```python
from build123d import *

# Parameters (mm, degrees)
F0_W     = 127
F0_H     = 127
F1_DEPTH = 12.7
F2_R     = 12.7
F3_DEPTH = 6.35
F4_R     = 1.5875
F5_DEPTH = 6.351


with BuildPart() as f1:
    # F0 (on Front) → F1 (new body)
    with BuildSketch(Plane.XZ):
        Rectangle(F0_W, F0_H)
    extrude(amount=F1_DEPTH)

    # F2 (on face) → F3 (cut)
    with BuildSketch(Plane.XZ.offset(12.7)):
        with Locations((0, 34.29)):
            Circle(F2_R)
        with Locations((-29.696011, -17.145)):
            Circle(F2_R)
        with Locations((29.696011, -17.145)):
            Circle(F2_R)
    extrude(amount=-F3_DEPTH, mode=Mode.SUBTRACT)

    # F4 (on face) → F5 (cut, through all)
    with BuildSketch(Plane.XZ.offset(6.35)):
        with Locations((0, 45.4025)):
            Circle(F4_R)
        with Locations((-39.319718, -22.70125)):
            Circle(F4_R)
        with Locations((39.319718, -22.70125)):
            Circle(F4_R)
    extrude(amount=-F5_DEPTH, mode=Mode.SUBTRACT)


solid = f1.part
```
The model under review builds one solid part; all positions refer to its coordinate system, in mm. A direction names the side the tool comes from. Coordinates: 2 decimals unless noted, no trailing zeros. Order: outer loops, then holes, each group sorted by start corner. A loop starts at its lowest first (then second) coordinate and runs counter-clockwise, first axis right, second up. Notation, with made-up numbers: (78.5, -14) -> (105.5, -14) arc R23 ccw to (105.5, 10) -> close; hole circle Ø1 at (-19.75, 80). An arc over 180 degrees is marked (long way). Answer in a Markdown table with one row per item. Add a question column.
Item 1: We need section A-A on z = 34.29. Write out the cut boundary in (x, y), plus the area to 3 significant figures.
Item 2: We need section C-C on x = 35. Write out the cut boundary in (y, z), plus the area to 3 significant figures.
Item 3: Machinability: for faces 1 (the flat face through (-30, -6.35, -17)), 2 (the cylindrical face through (-0.34, -3.22, 43.85)), which of the approach directions +Z, -Z, +X, -X, +Y, -Y give a long, thin tool a straight path to every point of the face, cutting with its end or side? Answer none if there is none.
Item 4: We need section B-B on y = -8.75. Write out the cut boundary in (x, z) (3 decimals), plus the area to 3 significant figures.
Item 5: Mouldability with a two-part tool opening along X and no side actions: class faces 3 (the flat face through (-1, -12.7, 1)), 4 (the cylindrical face through (-40.58, -3.219, -23.667)), 5 (the flat face through (0, -6.35, 34)), 6 (the flat face through (63.5, -6, -1)) as +X half, -X half, draft (parallel to the pull), parting line (faces both ways), or undercut.
Item 6: Clearance check with flat-ended pins moving along their axes: pin 1 (12.5 mm diameter, centred on x = 31, z = -14.5, fed in from -Y); pin 2 (1.9 mm diameter, centred on x = -39.32, z = -22.7, fed in from -Y). State where each tip first meets the part, or that it passes through.
Item 7: To check wall thickness, follow probe 1 along X at (y, z) = (-7, -16); probe 2 along Z at (x, y) = (0, -10.5); probe 3 along X at (y, z) = (-10.25, 34.29). State the ranges of each line that lie inside material, in increasing order.
Final values:
| question | item | result |
|---|---|---|
| 1 | outline | (-63.5, -12.7) -> (-12.7, -12.7) -> (-12.7, -6.35) -> (12.7, -6.35) -> (12.7, -12.7) -> (63.5, -12.7) -> (63.5, 0) -> (-63.5, 0) -> close |
| 1 | area | 1,450 mm2 |
| 2 | outline | (-12.7, -63.5) -> (0, -63.5) -> (0, 63.5) -> (-12.7, 63.5) -> (-12.7, -5.61) -> (-6.35, -5.61) -> (-6.35, -28.68) -> (-12.7, -28.68) -> close |
| 2 | area | 1,470 mm2 |
| 3 | face 1 | -Y |
| 3 | face 2 | +Y, -Y |
| 4 | outline | (-63.5, -63.5) -> (63.5, -63.5) -> (63.5, 63.5) -> (-63.5, 63.5) -> close; hole circle Ø25.4 at (-29.696, -17.145); hole circle Ø25.4 at (0, 34.29); hole circle Ø25.4 at (29.696, -17.145) |
| 4 | area | 14,600 mm2 |
| 5 | face 3 | draft |
| 5 | face 4 | undercut |
| 5 | face 5 | undercut |
| 5 | face 6 | +X half |
| 6 | pin 1 | stops at y = -6.35 |
| 6 | pin 2 | passes through |
| 7 | probe 1 | x = -63.5 to -42.34, -17.05 to 17.05, 42.34 to 63.5 |
| 7 | probe 2 | z = -63.5 to 21.59, 46.99 to 63.5 |
| 7 | probe 3 | x = -63.5 to -12.7, 12.7 to 63.5 |
